```python
from build123d import *

# Parameters (mm, degrees)
SKETCH1_R               = 1.5
SKETCH1_W               = 4
SKETCH1_H               = 80
BOSS_EXTRUDE1_DEPTH     = 10
CUT_EXTRUDE1_DEPTH      = 128.50847183
CUT_EXTRUDE1_DEPTH_BACK = 20
SKETCH2_R               = 2
SKETCH3_R               = 3
CUT_EXTRUDE2_DEPTH      = 20


with BuildPart() as part:
    # Sketch1 → Boss-Extrude1 (new body)
    with BuildSketch(Plane.XY):
        with BuildLine():
            Line((-85, -85), (-85, -65))
            Line((-85, -65), (-44.1, -65))
            Line((-44.1, -65), (-44.1, -85))
            ThreePointArc((-44.1, -85), (-40.1, -86.656854249), (-36.1, -85))
            Line((-36.1, -85), (-36.1, -60))
            ThreePointArc((-36.1, -60), (0, -45.046890398), (36.1, -60))
            Line((36.1, -60), (36.1, -85))
            ThreePointArc((36.1, -85), (40.1, -86.656854249), (44.1, -85))
            Line((44.1, -85), (44.1, -65))
            Line((44.1, -65), (85, -65))
            Line((85, -65), (85, -85))
            ThreePointArc((85, -85), (89, -86.656854249), (93, -85))
            Line((93, -85), (93, -60))
            ThreePointArc((93, -60), (68.147186258, 0), (93, 60))
            Line((93, 60), (93, 85))
            ThreePointArc((93, 85), (89, 86.656854249), (85, 85))
            Line((85, 85), (85, 65))
            Line((85, 65), (44.1, 65))
            Line((44.1, 65), (44.1, 85))
            ThreePointArc((44.1, 85), (40.1, 86.656854249), (36.1, 85))
            Line((36.1, 85), (36.1, 60))
            ThreePointArc((36.1, 60), (0, 45.046890398), (-36.1, 60))
            Line((-36.1, 60), (-36.1, 85))
            ThreePointArc((-36.1, 85), (-40.1, 86.656854249), (-44.1, 85))
            Line((-44.1, 85), (-44.1, 65))
            Line((-44.1, 65), (-85, 65))
            Line((-85, 65), (-85, 85))
            ThreePointArc((-85, 85), (-89, 86.656854249), (-93, 85))
            Line((-93, 85), (-93, 60))
            ThreePointArc((-93, 60), (-68.147186258, 0), (-93, -60))
            Line((-93, -60), (-93, -85))
            ThreePointArc((-93, -85), (-89, -86.656854249), (-85, -85))
        make_face()
        with Locations((-89, 70)):
            Circle(SKETCH1_R, mode=Mode.SUBTRACT)
        with Locations((-89, 80)):
            Circle(SKETCH1_R, mode=Mode.SUBTRACT)
        with Locations((-40.1, 70)):
            Circle(SKETCH1_R, mode=Mode.SUBTRACT)
        with Locations((-40.1, 80)):
            Circle(SKETCH1_R, mode=Mode.SUBTRACT)
        with Locations((-40.1, -70)):
            Circle(SKETCH1_R, mode=Mode.SUBTRACT)
        with Locations((-40.1, -80)):
            Circle(SKETCH1_R, mode=Mode.SUBTRACT)
        with Locations((-89, -80)):
            Circle(SKETCH1_R, mode=Mode.SUBTRACT)
        with Locations((-89, -70)):
            Circle(SKETCH1_R, mode=Mode.SUBTRACT)
        with Locations((89, 80)):
            Circle(SKETCH1_R, mode=Mode.SUBTRACT)
        with Locations((89, 70)):
            Circle(SKETCH1_R, mode=Mode.SUBTRACT)
        with Locations((40.1, 80)):
            Circle(SKETCH1_R, mode=Mode.SUBTRACT)
        with Locations((40.1, 70)):
            Circle(SKETCH1_R, mode=Mode.SUBTRACT)
        with Locations((89, -70)):
            Circle(SKETCH1_R, mode=Mode.SUBTRACT)
        with Locations((89, -80)):
            Circle(SKETCH1_R, mode=Mode.SUBTRACT)
        with Locations((40.1, -80)):
            Circle(SKETCH1_R, mode=Mode.SUBTRACT)
        with Locations((40.1, -70)):
            Circle(SKETCH1_R, mode=Mode.SUBTRACT)
        with Locations((44.1, 0)):
            Rectangle(SKETCH1_W, SKETCH1_H, mode=Mode.SUBTRACT)
        with Locations((-44.1, 0)):
            Rectangle(SKETCH1_W, SKETCH1_H, mode=Mode.SUBTRACT)
        Rectangle(SKETCH1_W, SKETCH1_H, mode=Mode.SUBTRACT)
    extrude(amount=BOSS_EXTRUDE1_DEPTH)

    # Sketch2 → Cut-Extrude1 (cut, two sides: drawn at the far end of the back side and taken through both)
    with BuildSketch(Plane.XY.offset(10).offset(-CUT_EXTRUDE1_DEPTH_BACK)):
        with Locations(Location((53.15, -48.68, 0), (0, 0, 180))):
            Circle(SKETCH2_R)
        with Locations(Location((-53.15, -48.68, 0), (0, 0, 180))):
            Circle(SKETCH2_R)
        with Locations(Location((53.15, 48.68, 0), (0, 0, 180))):
            Circle(SKETCH2_R)
        with Locations(Location((-53.15, 48.68, 0), (0, 0, 180))):
            Circle(SKETCH2_R)
    extrude(amount=CUT_EXTRUDE1_DEPTH + CUT_EXTRUDE1_DEPTH_BACK, mode=Mode.SUBTRACT)

    # Sketch3 → Cut-Extrude2 (cut)
    with BuildSketch(Plane.XY.offset(10)):
        with Locations((18, 0)):
            Circle(SKETCH3_R)
        with Locations((-18, 0)):
            Circle(SKETCH3_R)
    extrude(amount=-CUT_EXTRUDE2_DEPTH, mode=Mode.SUBTRACT)


solid = part.part
```
Source: CAD feature listing. Evaluate the final solid. Frame: model axes, mm. A direction names the side the tool comes from. Coordinates: 2 decimals unless noted, no trailing zeros. Order: outer loops, then holes, each group sorted by start corner. A loop starts at its lowest first (then second) coordinate and runs counter-clockwise, first axis right, second up. Notation, with made-up numbers: (18.25, 17.25) - (29.25, 17.25) arc R30 cw to (29.25, 39.25) - close; hole circle Ø4 at (88.5, 81). An arc over 180 degrees is marked (long way). One line per item, written item: value.
1) Cut plane D-D on y = 31. Output: boundary loops of the cut face in (x, z).
Computed values:
outline: (-74.01, 0) - (-46.1, 0) - (-46.1, 10) - (-74.01, 10) - close; (-42.1, 0) - (-2, 0) - (-2, 10) - (-42.1, 10) - close; (2, 0) - (42.1, 0) - (42.1, 10) - (2, 10) - close; (46.1, 0) - (74.01, 0) - (74.01, 10) - (46.1, 10) - close
2) Mould query, pull axis X, two halves, no side actions, for faces 4 (the face through (68.152, -0.933, 4.93)), 5 (the face through (-68.152, 0.933, 4.93)), 6 (the face through (65, 65, 5)). Classes: released by +X, released by -X, zero draft, split by the parting line, or undercut.
Computed values:
face 4: released by +X
face 5: released by -X
face 6: undercut
3) Reachability of faces 1 (the face through (-42.1, -1, 5)), 2 (the face through (44.1, -75, 5)), 3 (the face through (36.1, 73, 5)) from +Z, -Z, +X, -X, +Y, -Y: full face, straight path, thin tool, end or side. Return the list, or none.
Computed values:
face 1: +Z, -Z
face 2: +Z, -Z, -Y
face 3: +Z, -Z, +Y
4) Contact query for flat-ended pins moving along their axis: pin 1 (3 mm diameter, centred on x = 44.5, z = 5, fed in from +Y); pin 2 (7 mm diameter, centred on x = -18, y = 0, fed in from +Z); pin 3 (4.5 mm diameter, centred on x = -44, z = 7.5, fed in from +Y); pin 4 (3 mm diameter, centred on y = 9.5, z = 4.5, fed in from -X). Output: stop coordinate, or through.
Computed values:
pin 1: stops at y = 85.86
pin 2: stops at z = 10
pin 3: stops at y = 86.41
pin 4: stops at x = -68.86
5) Ray query, line 1 (Y direction, x = -53.15, z = 7.75); line 2 (Y direction, x = 89, z = 4.75); line 3 (X direction, y = 3.5, z = 4.75). Return the intervals inside material, ascending. Write a range as [from, to].
Computed values:
line 1: y = [-65, -50.68], [-46.68, 46.68], [50.68, 65]
line 2: y = [-86.66, -81.5], [-78.5, -71.5], [-68.5, -55.71], [55.71, 68.5], [71.5, 78.5], [81.5, 86.66]
line 3: x = [-68.22, -46.1], [-42.1, -2], [2, 42.1], [46.1, 68.22]
6) Cut plane B-B on y = -17.5. Output: boundary loops of the cut face in (x, z), plus the area to 3 significant figures.
Computed values:
outline: (-69.97, 0) - (-46.1, 0) - (-46.1, 10) - (-69.97, 10) - close; (-42.1, 0) - (-2, 0) - (-2, 10) - (-42.1, 10) - close; (2, 0) - (42.1, 0) - (42.1, 10) - (2, 10) - close; (46.1, 0) - (69.97, 0) - (69.97, 10) - (46.1, 10) - close
area: 1,280 mm^2
7) Cut plane A-A on y = 0. Output: boundary loops of the cut face in (x, z), plus the area to 3 significant figures.
Computed values:
outline: (-68.15, 0) - (-46.1, 0) - (-46.1, 10) - (-68.15, 10) - close; (-42.1, 0) - (-21, 0) - (-21, 10) - (-42.1, 10) - close; (-15, 0) - (-2, 0) - (-2, 10) - (-15, 10) - close; (2, 0) - (15, 0) - (15, 10) - (2, 10) - close; (21, 0) - (42.1, 0) - (42.1, 10) - (21, 10) - close; (46.1, 0) - (68.15, 0) - (68.15, 10) - (46.1, 10) - close
area: 1,120 mm^2
8) Cut plane C-C on z = 6. State how many separate pieces and enclosed holes the cut face has, plus the area to 3 significant figures.
Computed values:
separate pieces: 1
enclosed holes: 25
area: 18,000 mm^2
